Solid Edge part; units mm, degrees
sketch "Sketch1" plane through (0, 0, 0) normal (0, -1, 0) x (1, 0, 0)
  line L0 (-50, 0) -> (-50, 7.5)
  line L1 (-50, 7.5) -> (-21, 7.5)
  line L2 (-21, 7.5) -> (-21, 6.5)
  line L3 (-21, 6.5) -> (-19, 6.5)
  line L4 (-19, 6.5) -> (-19, 9)
  line L5 (-19, 9) -> (19, 9)
  line L6 (19, 9) -> (19, 6.5)
  line L7 (19, 6.5) -> (21, 6.5)
  line L8 (21, 6.5) -> (21, 7.5)
  line L9 (21, 7.5) -> (50, 7.5)
  line L10 (50, 7.5) -> (50, 0)
  dimension "D1" = 50
  dimension "D2" = 19
  dimension "D3" = 21
revolve "RevolvedProtrusion1" add sketch "Sketch1" angle 360 about axis through (50, 0, 0) along (-1, 0, 0)
chamfer "Chamfer1" distance 0.5 angle 45 4 edges at (-50, 0, -7.5) (50, 0, -7.5) (-19, 0, -9) (19, 0, -9)
fillet "Round_1" radius 1 4 edges at (-21, 0, -6.5) (-19, 0, -6.5) (19, 0, -6.5) (21, 0, -6.5)
properties material "AlSi7Mg"
Input: part model. Units: mm. Frame: model coordinates. A direction names the side the tool comes from. Round coordinates to 2 decimals unless told otherwise and drop trailing zeros. Order: outer loops, then holes, each group sorted by start corner. A loop starts at its lowest first (then second) coordinate and runs counter-clockwise, first axis right, second up. Notation, with made-up numbers: (27, 41) - (55, 41) arc R9 ccw to (55, 45) - close; hole circle Ø1 at (58, 44). An arc over 180 degrees is marked (long way). Answer in a Markdown table with one row per item.
Item 1: Pin query (flat end, axial travel): pin 1 (6 mm diameter, centred on x = -24.5, y = 6, fed in from +Z); pin 2 (5 mm diameter, centred on x = 17, y = 7, fed in from -Z); pin 3 (4 mm diameter, centred on x = 12.5, y = -7, fed in from -Z). Return the tip coordinate at first contact, or that it passes through.
Model answer:
| item | result |
|---|---|
| pin 1 | stops at z = 6.87 |
| pin 2 | stops at z = -7.79 |
| pin 3 | stops at z = -7.48 |
Item 2: Line query: line 1 (X direction, y = 7, z = 0.5); line 2 (X direction, y = -3.25, z = -6); line 3 (X direction, y = -6, z = -5). Output: solid intervals per line, ascending.
Model answer:
| item | result |
|---|---|
| line 1 | x = -49.98 to -20.88, -19.12 to 19.12, 20.88 to 49.98 |
| line 2 | x = -50 to -20.74, -19.26 to 19.26, 20.74 to 50 |
| line 3 | x = -19 to 19 |
Item 3: Section query A-A (x = -17). Return the cut outline in (y, z), then the cut area to 3 significant figures.
Model answer:
| item | result |
|---|---|
| outline | circle Ø18 at (0, 0) |
| area | 254 mm² |
Item 4: Reachability of faces 1 (the flat face through (19, -8, 0)), 2 (the cylindrical face through (-35.05, -0.33, -7.493)), 3 (the flat face through (50, 0, 0)) from +Z, -Z, +X, -X, +Y, -Y: full face, straight path, thin tool, end or side. Return the list, or none.
Model answer:
| item | result |
|---|---|
| face 1 | +X |
| face 2 | -X |
| face 3 | +Z, -Z, +X, +Y, -Y |
Item 5: Section query B-B (x = -29.5). Return the cut outline in (y, z).
Model answer:
| item | result |
|---|---|
| outline | circle Ø15 at (0, 0) |
